Check sheet for the modelled part. Datum: model origin and axes. Units: mm. A direction names the side the tool comes from. Give positions to 0.01 mm unless a question says otherwise; leave off trailing zeros. Loops run counter-clockwise (first coordinate to the right, second up) from the corner with the lowest first, then second, coordinate; pieces in that order, holes last. Notation, with made-up numbers: (-15, 42.5) - (30, 42.5) arc R7 ccw to (30, 53.5) - close; hole circle Ø2 at (14.25, -10.75). An arc over 180 degrees is marked (long way). Answer in a Markdown table with one row per item. Add a question column.
(1) Thickness scan on L1, parallel to Y at x = -1, z = 0 (3 decimals); L2, parallel to X at y = -6, z = 5; L3, parallel to Y at x = 3.75, z = 0. Record the ranges inside material, lowest first.
(2) Sectioned sample at C-C on x = -1. Enter the section's corners in (y, z) (3 decimals).
(3) Go/stop test with flat-tipped pins: P1, Ø1.5, axis at x = -5, z = 6, coming from the -Y side; P2, Ø1, axis at x = 4, y = 3, coming from the +Z side; P3, Ø4, axis at y = 0, z = 0, coming from the -X side; P4, Ø3, axis at x = -4.5, y = -5.5, coming from the -Z side. Record where each tip stops, or that it passes through.
(4) Sectioned sample at B-B on x = 4. Enter the section's corners in (y, z), then the cut area to 3 significant figures.
(5) Sectioned sample at A-A on z = 0. Enter the section's corners in (x, y) (1 decimal), then the cut area to 3 significant figures.
(6) Set-up check for faces 1 (the face through (-1.651, 6, -2)), 2 (the face through (-4.115, -9.546, 2.12)): record each of +Z, -Z, +X, -X, +Y, -Y from which the full face is reachable in a straight line by a thin tool's end or side.
(7) Draft check along X on faces 3 (the face through (-6.604, 2, -2)), 4 (the face through (1.651, 6, -2)), 5 (the face through (4.14, -9.546, 2.12)), 6 (the face through (6.604, 2, -2)). Enter one of: released by +X, released by -X, zero draft, split by the parting line, or undercut.
from build123d import *

# Parameters (mm, degrees)
SKETCH1_R           = 9.779
SKETCH1_R_2         = 2.5
BOSS_EXTRUDE1_DEPTH = 6.604
SKETCH2_R           = 11.049
SKETCH2_R_2         = 5.675
CUT_EXTRUDE1_DEPTH  = 1.651
FILLET1_R           = 1.5875


with BuildPart() as part:
    # Sketch1 → Boss-Extrude1 (new body, symmetric)
    with BuildSketch(Plane(origin=(0, 0, 0), x_dir=(0, 0, -1), z_dir=(1, 0, 0))):
        Circle(SKETCH1_R)
        Circle(SKETCH1_R_2, mode=Mode.SUBTRACT)
    extrude(amount=BOSS_EXTRUDE1_DEPTH, both=True)

    # Sketch2 → Cut-Extrude1 (cut, symmetric)
    with BuildSketch(Plane(origin=(0, 0, 0), x_dir=(0, 0, -1), z_dir=(1, 0, 0))):
        Circle(SKETCH2_R)
        Circle(SKETCH2_R_2, mode=Mode.SUBTRACT)
    extrude(amount=CUT_EXTRUDE1_DEPTH, both=True, mode=Mode.SUBTRACT)

    # Fillet1
    fillet1_edges = [part.edges().sort_by_distance(p)[0] for p in [
        (1.651, 0, 9.779),
        (-1.651, 0, 9.779),
        (-6.604, 0, 9.779),
        (6.604, 0, 9.779),
    ]]
    fillet(fillet1_edges, radius=FILLET1_R)


solid = part.part
Reply:
| question | item | result |
|---|---|---|
| 1 | L1 | -5.675 to -2.5, 2.5 to 5.675 |
| 1 | L2 | -6.6 to -1.65, 1.65 to 6.6 |
| 1 | L3 | -9.78 to -2.5, 2.5 to 9.78 |
| 2 | outline | circle Ø11.35 at (0, 0); hole circle Ø5 at (0, 0) |
| 3 | P1 | y = -8.25 |
| 3 | P2 | z = 9.45 |
| 3 | P3 | through |
| 3 | P4 | z = -8.92 |
| 4 | outline | circle Ø19.56 at (0, 0); hole circle Ø5 at (0, 0) |
| 4 | area | 281 mm^2 |
| 5 | outline | (-6.6, -8.2) arc R1.6 ccw to (-5, -9.8) - (-3.2, -9.8) arc R1.6 ccw to (-1.7, -8.2) - (-1.7, -5.7) - (1.7, -5.7) - (1.7, -8.2) arc R1.6 ccw to (3.2, -9.8) - (5, -9.8) arc R1.6 ccw to (6.6, -8.2) - (6.6, -2.5) - (-6.6, -2.5) - close; (-6.6, 2.5) - (6.6, 2.5) - (6.6, 8.2) arc R1.6 ccw to (5, 9.8) - (3.2, 9.8) arc R1.6 ccw to (1.7, 8.2) - (1.7, 5.7) - (-1.7, 5.7) - (-1.7, 8.2) arc R1.6 ccw to (-3.2, 9.8) - (-5, 9.8) arc R1.6 ccw to (-6.6, 8.2) - close |
| 5 | area | 161 mm^2 |
| 6 | face 1 | none |
| 6 | face 2 | +X, -X |
| 7 | face 3 | released by -X |
| 7 | face 4 | undercut |
| 7 | face 5 | zero draft |
| 7 | face 6 | released by +X |
